```python
from build123d import *

# Parameters (mm, degrees)
SKIZZE1_W                        = 35
SKIZZE1_H                        = 75
AUFSATZ_LINEAR_AUSTRAGEN1_DEPTH  = 1.5
SKIZZE3_W                        = 15.25
SKIZZE3_H                        = 5
SKIZZE3_W_2                      = 4.875
SCHNITT_LINEAR_AUSTRAGEN12_DEPTH = 20
SCHNITT_LINEAR_AUSTRAGEN14_DEPTH = 1.5
VERRUNDUNG1_R                    = 10
VERRUNDUNG2_R                    = 10


with BuildPart() as part:
    # Skizze1 → Aufsatz-Linear austragen1 (new body)
    with BuildSketch(Plane.XY):
        with Locations((17.5, 37.5)):
            Rectangle(SKIZZE1_W, SKIZZE1_H)
    extrude(amount=AUFSATZ_LINEAR_AUSTRAGEN1_DEPTH)

    # Skizze3 → Schnitt-Linear austragen12 (cut)
    with BuildSketch(Plane.XY.offset(1.5)):
        with Locations((17.5, 2.5)):
            Rectangle(SKIZZE3_W, SKIZZE3_H)
        with Locations((32.5625, 2.5)):
            Rectangle(SKIZZE3_W_2, SKIZZE3_H)
        with Locations((2.4375, 2.5)):
            Rectangle(SKIZZE3_W_2, SKIZZE3_H)
    extrude(amount=-SCHNITT_LINEAR_AUSTRAGEN12_DEPTH, mode=Mode.SUBTRACT)

    # Skizze7 → Schnitt-Linear austragen14 (cut)
    with BuildSketch(Plane.XY.offset(1.5)):
        with BuildLine():
            Line((29.980893063, 50.823094237), (5.5, 18))
            Line((5.5, 18), (5.5, 17))
            Line((5.5, 17), (29.5, 17))
            Line((29.5, 17), (29.5, 18))
            Line((29.5, 18), (6.7, 18))
            Line((6.7, 18), (30.963924784, 50.532191031))
            ThreePointArc((30.963924784, 50.532191031), (20.317920223, 64.291686591), (5.520765623, 55.142623967))
            Line((5.520765623, 55.142623967), (6.566221507, 55.142623967))
            ThreePointArc((6.566221507, 55.142623967), (20.177020409, 63.300872092), (29.980893063, 50.823094237))
        make_face()
    extrude(amount=-SCHNITT_LINEAR_AUSTRAGEN14_DEPTH, mode=Mode.SUBTRACT)

    # Verrundung1
    verrundung1_edges = [part.edges().sort_by_distance(p)[0] for p in [
        (30.963924784, 50.532191031, 0.75),
    ]]
    fillet(verrundung1_edges, radius=VERRUNDUNG1_R)

    # Verrundung2
    verrundung2_edges = [part.edges().sort_by_distance(p)[0] for p in [
        (29.980893063, 50.823094237, 0.75),
    ]]
    fillet(verrundung2_edges, radius=VERRUNDUNG2_R)


solid = part.part
```
Build history of the part. All positions in model axes, mm. A direction names the side the tool comes from. Give positions to 0.01 mm unless a question says otherwise; leave off trailing zeros. Loops run counter-clockwise (first coordinate to the right, second up) from the corner with the lowest first, then second, coordinate; pieces in that order, holes last. Notation, with made-up numbers: (-40, 1) - (-11, 1) arc R9 cw to (-11, 8) - close; hole circle Ø11 at (-37.75, 83). An arc over 180 degrees is marked (long way). Use a Markdown table: item, result.
(1) Band-saw the part on B-B (z = 0.8). Give the cut face in (x, y) (3 decimals), and give its area (3 significant figures).
Taken from the geometry:
| item | result |
|---|---|
| outline | (0, 5) - (4.875, 5) - (4.875, 0) - (9.875, 0) - (9.875, 5) - (25.125, 5) - (25.125, 0) - (30.125, 0) - (30.125, 5) - (35, 5) - (35, 75) - (0, 75) - close; hole (5.5, 17) - (29.5, 17) - (29.5, 18) - (6.7, 18) - (28.491, 47.217) arc R10 ccw to (28.725, 58.846) arc R13 ccw to (5.521, 55.143) - (6.566, 55.143) arc R12 cw to (25.215, 61.088) arc R10 cw to (27.219, 47.119) - (5.5, 18) - close |
| area | 2,400 mm2 |
(2) Band-saw the part on C-C (x = 16). Give the cut face in (y, z), and give its area (3 significant figures).
Taken from the geometry:
| item | result |
|---|---|
| outline | (5, 0) - (17, 0) - (17, 1.5) - (5, 1.5) - close; (18, 0) - (30.47, 0) - (30.47, 1.5) - (18, 1.5) - close; (32.08, 0) - (63.33, 0) - (63.33, 1.5) - (32.08, 1.5) - close; (64.35, 0) - (75, 0) - (75, 1.5) - (64.35, 1.5) - close |
| area | 99.6 mm2 |
(3) Band-saw the part on A-A (y = 20). Give the cut face in (x, z), and give its area (3 significant figures).
Taken from the geometry:
| item | result |
|---|---|
| outline | (0, 0) - (6.99, 0) - (6.99, 1.5) - (0, 1.5) - close; (8.19, 0) - (35, 0) - (35, 1.5) - (8.19, 1.5) - close |
| area | 50.7 mm2 |
(4) Pull direction Y, two halves, no side cores. Call faces 6 (the face through (35, 40, 1)), 7 (the face through (7, 0, 1)), 8 (the face through (17, 17, 1)): +Y half, -Y half, draft (parallel to the pull), parting line (faces both ways), or undercut.
Taken from the geometry:
| item | result |
|---|---|
| face 6 | draft |
| face 7 | -Y half |
| face 8 | undercut |
(5) Which spindle directions (+Z, -Z, +X, -X, +Y, -Y) get a long thin tool onto all of the face, cutting with end or side? Do faces 1 (the face through (17, 5, 1)), 2 (the face through (28, 0, 1)), 3 (the face through (30.125, 2, 1)), 4 (the face through (17.44, 32.4, 0.76)), 5 (the face through (4.875, 2, 1)). Say none if no direction does.
Taken from the geometry:
| item | result |
|---|---|
| face 1 | +Z, -Z, -Y |
| face 2 | +Z, -Z, +X, -X, -Y |
| face 3 | +Z, -Z, +X, -Y |
| face 4 | +Z, -Z |
| face 5 | +Z, -Z, -X, -Y |
(6) Band-saw the part on D-D (x = 23). Give the cut face in (y, z).
Taken from the geometry:
| item | result |
|---|---|
| outline | (5, 0) - (17, 0) - (17, 1.5) - (5, 1.5) - close; (18, 0) - (39.85, 0) - (39.85, 1.5) - (18, 1.5) - close; (41.46, 0) - (62.41, 0) - (62.41, 1.5) - (41.46, 1.5) - close; (63.5, 0) - (75, 0) - (75, 1.5) - (63.5, 1.5) - close |
(7) Wall check: line 1 along X through (y, z) = (58, 0.3); line 2 along Y through (x, z) = (26, 1.1); line 3 along Y through (x, z) = (9.5, 0.75). Give the ranges that are in metal, low to high.
Taken from the geometry:
| item | result |
|---|---|
| line 1 | 0 to 6.74, 7.91 to 27.92, 29.25 to 35 |
| line 2 | 0 to 17, 18 to 43.88, 45.49 to 60.43, 61.75 to 75 |
| line 3 | 0 to 17, 18 to 21.75, 23.36 to 59.97, 61.34 to 75 |
(8) Drop flat-ended pins along their axis: pin 1 Ø3 at (x, y) = (31, 49.5) entering from -Z; pin 2 Ø0.8 at (y, z) = (3.5, 0.5) entering from +X (3 decimals); pin 3 Ø0.8 at (x, z) = (22, 1) entering from -Y; pin 4 Ø0.8 at (y, z) = (2, 1) entering from -X (3 decimals). Give the stop position or say it passes through.
Taken from the geometry:
| item | result |
|---|---|
| pin 1 | z = 0 |
| pin 2 | x = 30.125 |
| pin 3 | y = 5 |
| pin 4 | x = 4.875 |
